Verification items for the finished model (mm, model axes). Give positions to 0.01 mm unless a question says otherwise; leave off trailing zeros. Loops run counter-clockwise (first coordinate to the right, second up) from the corner with the lowest first, then second, coordinate; pieces in that order, holes last. Notation, with made-up numbers: M 16,-33 L 34,-33 A26 ccw 34,-9 Z; hole C 38,72 d3. An arc over 180 degrees is marked long. Write each question's results on one line, items separated by ' | '. Start each with the question number.
```python
from build123d import *

# Parameters (mm, degrees)
SKETCH1_W           = 63.5
SKETCH1_H           = 63.5
SKETCH1_R           = 6.35
BOSS_EXTRUDE1_DEPTH = 19.05
SKETCH3_R           = 4.4958
CUT_EXTRUDE2_DEPTH  = 19.05


with BuildPart() as part:
    # Sketch1 → Boss-Extrude1 (new body)
    with BuildSketch(Plane(origin=(0, 0, 0), x_dir=(1, 0, 0), z_dir=(0, 1, 0))):
        with Locations((-4.445666472, -11.8618)):
            Rectangle(SKETCH1_W, SKETCH1_H)
        with Locations(Location((-4.445666472, -11.8618, 0), (0, 0, 90))):
            Circle(SKETCH1_R, mode=Mode.SUBTRACT)
    extrude(amount=BOSS_EXTRUDE1_DEPTH)

    # Sketch3 → Cut-Extrude2 (cut)
    with BuildSketch(Plane(origin=(0, 0, 0), x_dir=(1, 0, 0), z_dir=(0, 1, 0))):
        with Locations(Location((-24.448166472, 8.1407, 0), (0, 0, 90))):
            Circle(SKETCH3_R)
        with Locations(Location((15.556833528, 8.1407, 0), (0, 0, 90))):
            Circle(SKETCH3_R)
        with Locations(Location((15.556833528, -31.8643, 0), (0, 0, 90))):
            Circle(SKETCH3_R)
        with Locations(Location((-24.448166472, -31.8643, 0), (0, 0, 90))):
            Circle(SKETCH3_R)
    extrude(amount=CUT_EXTRUDE2_DEPTH, mode=Mode.SUBTRACT)


solid = part.part
```
1. Section check B-B, the plane x = -10. Record the boundary of the cut face in (y, z).
2. Thickness scan on probe 1 along X at (y, z) = (8, -8); probe 2 along Z at (x, y) = (14, 15.75); probe 3 along Z at (x, y) = (19.5, 6.25). Record the ranges inside material, lowest first.
3. Section check C-C, the plane y = 10. Record the boundary of the cut face in (x, z), plus the area to 3 significant figures.
4. Section check A-A, the plane z = 13. Record the boundary of the cut face in (x, y).
5. Release check for a two-part mould opening along Z. For faces 1 (the face through (11.766, 9.392, 29.447)), 2 (the face through (-36.196, 9, 12)), 3 (the face through (-5, 9, 43.612)) record: released by +Z, released by -Z, zero draft, split by the parting line, or undercut.
6. Section check D-D, the plane z = -6. Record the boundary of the cut face in (x, y), plus the area to 3 significant figures.
Filled sheet:
1) outline: M 0,-19.89 L 19.05,-19.89 L 19.05,8.78 L 0,8.78 Z; M 0,14.94 L 19.05,14.94 L 19.05,43.61 L 0,43.61 Z
2) probe 1: -36.2 to -28.94, -19.95 to 11.06, 20.05 to 27.3 | probe 2: -19.89 to -12.36, -3.92 to 27.65, 36.08 to 43.61 | probe 3: -19.89 to -10.3, -5.98 to 29.7, 34.02 to 43.61
3) outline: M -36.2,-19.89 L 27.3,-19.89 L 27.3,43.61 L -36.2,43.61 Z; hole C -24.45,-8.14 d8.99; hole C -24.45,31.86 d8.99; hole C -4.45,11.86 d12.7; hole C 15.56,-8.14 d8.99; hole C 15.56,31.86 d8.99 | area: 3,650 mm2
4) outline: M -36.2,0 L -10.69,0 L -10.69,19.05 L -36.2,19.05 Z; M 1.8,0 L 27.3,0 L 27.3,19.05 L 1.8,19.05 Z
5) face 1: undercut | face 2: zero draft | face 3: released by +Z
6) outline: M -36.2,0 L -28.4,0 L -28.4,19.05 L -36.2,19.05 Z; M -20.49,0 L 11.6,0 L 11.6,19.05 L -20.49,19.05 Z; M 19.51,0 L 27.3,0 L 27.3,19.05 L 19.51,19.05 Z | area: 908 mm2
